Source: three-view drawing plus pictorial views. Frame: mm from the lowest corner of the part. A direction names the side the tool comes from. Give positions to 0.01 mm unless a question says otherwise; leave off trailing zeros. Order: outer loops, then holes, each group sorted by start corner. A loop starts at its lowest first (then second) coordinate and runs counter-clockwise, first axis right, second up. Notation, with made-up numbers: (-7, -11) - (8, -11) arc R19 ccw to (8, 20) - close; hole circle Ø4 at (29, -5.5). An arc over 180 degrees is marked (long way). Use CSV: the item, a comma, the result in double quotes.
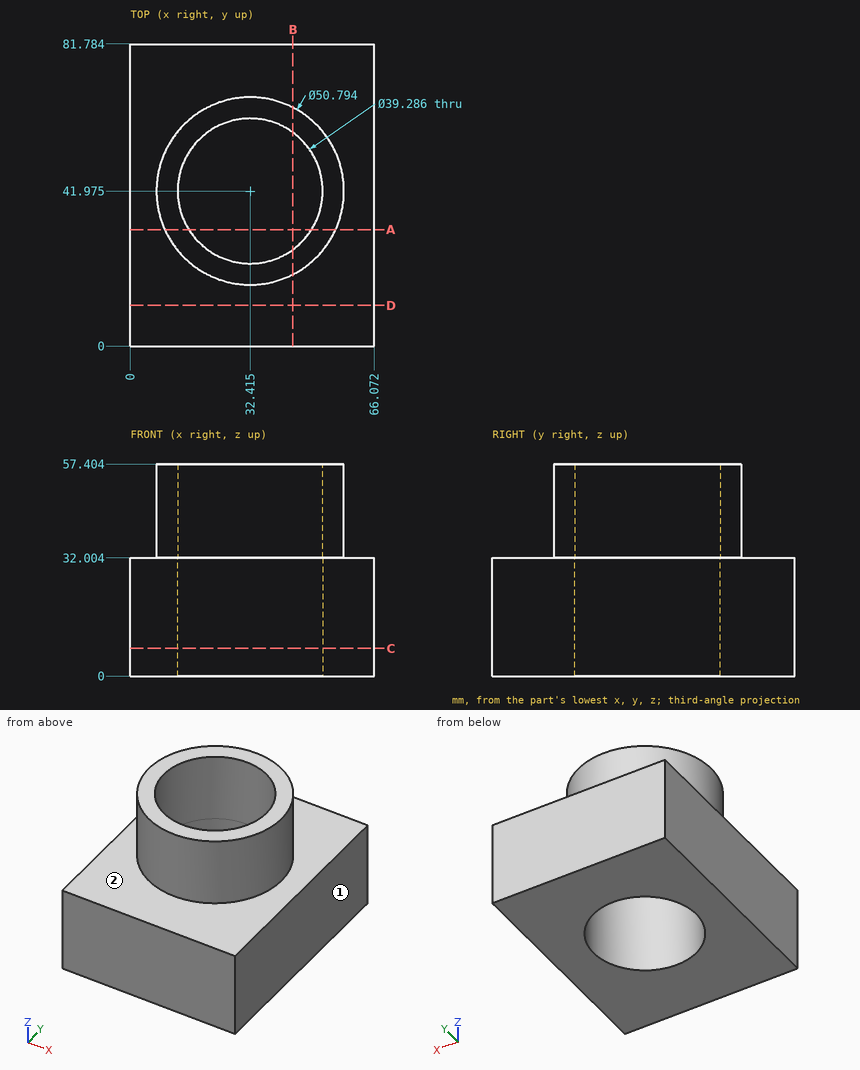
Item 1: Section C-C on z = 7.5. Return the cut outline in (x, y) (1 decimal), then the cut area to 3 significant figures.
Filled in:
outline,"(0, 0) - (66.1, 0) - (66.1, 81.8) - (0, 81.8) - close; hole circle Ø39.3 at (32.4, 42)"
area,"4,190 mm2"
Item 2: Section B-B on x = 44. Return the cut outline in (y, z) (1 decimal), then the cut area to 3 significant figures.
Filled in:
outline,"(0, 0) - (26.1, 0) - (26.1, 57.4) - (19.4, 57.4) - (19.4, 32) - (0, 32) - close; (57.8, 0) - (81.8, 0) - (81.8, 32) - (64.6, 32) - (64.6, 57.4) - (57.8, 57.4) - close"
area,"1,940 mm2"
Item 3: Set-up query: the marked faces 1 and 2. Return all of +Z, -Z, +X, -X, +Y, -Y with unobstructed straight access to the full face (end or side cutting, diameter ignored); none if empty.
Filled in:
face 1,"+Z, -Z, +X, +Y, -Y"
face 2,"+Z"
Item 4: Section D-D on y = 11. Return the cut outline in (x, z) (1 decimal).
Filled in:
outline,"(0, 0) - (66.1, 0) - (66.1, 32) - (0, 32) - close"
Item 5: First-contact query: pin 1 (6 mm diameter, centred on x = 28, z = 44.5, fed in from -Y); pin 2 (8 mm diameter, centred on x = 51, y = 10.5, fed in from +Z). Flat tips, straight axial feed; report the tip coordinate or a pass-through.
Filled in:
pin 1,"stops at y = 16.62"
pin 2,"stops at z = 32"
Item 6: Section A-A on y = 31.5. Return the cut outline in (x, z) (1 decimal).
Filled in:
outline,"(0, 0) - (15.8, 0) - (15.8, 57.4) - (9.3, 57.4) - (9.3, 32) - (0, 32) - close; (49, 0) - (66.1, 0) - (66.1, 32) - (55.6, 32) - (55.6, 57.4) - (49, 57.4) - close"
Item 7: Material intervals for line 1 (Y direction, x = 22.5, z = 4.5) (1 decimal); line 2 (X direction, y = 32, z = 21) (1 decimal); line 3 (X direction, y = 26, z = 10) (1 decimal), sorted ascending. Write a range as from..to.
Filled in:
line 1,"y = 0..25, 58.9..81.8"
line 2,"x = 0..15.5, 49.3..66.1"
line 3,"x = 0..21, 43.8..66.1"
